from build123d import *

# Parameters (mm, degrees)
SKETCH1_W           = 50
SKETCH1_H           = 57
BOSS_EXTRUDE1_DEPTH = 52
SKETCH2_W           = 18
SKETCH2_H           = 50
CUT_EXTRUDE1_DEPTH  = 52
SKETCH3_W           = 8
SKETCH3_H           = 50
CUT_EXTRUDE2_DEPTH  = 52
SKETCH4_R           = 15
SKETCH4_R_2         = 7
BOSS_EXTRUDE2_DEPTH = 30


with BuildPart() as part:
    # Sketch1 → Boss-Extrude1 (new body)
    with BuildSketch(Plane.XY):
        with Locations((25, 28.5)):
            Rectangle(SKETCH1_W, SKETCH1_H)
    extrude(amount=-BOSS_EXTRUDE1_DEPTH)

    # Sketch2 → Cut-Extrude1 (cut)
    with BuildSketch(Plane.XY):
        with Locations((25, 25)):
            Rectangle(SKETCH2_W, SKETCH2_H)
    extrude(amount=-CUT_EXTRUDE1_DEPTH, mode=Mode.SUBTRACT)

    # Sketch3 → Cut-Extrude2 (cut)
    with BuildSketch(Plane.XY):
        with Locations((46, 32)):
            Rectangle(SKETCH3_W, SKETCH3_H)
        with Locations((4, 32)):
            Rectangle(SKETCH3_W, SKETCH3_H)
    extrude(amount=-CUT_EXTRUDE2_DEPTH, mode=Mode.SUBTRACT)

    # Sketch4 → Boss-Extrude2 (add)
    with BuildSketch(Plane(origin=(42, 0, 0), x_dir=(0, 0, -1), z_dir=(1, 0, 0))):
        with Locations(Location((26, 33, 0), (0, 0, 180))):
            Circle(SKETCH4_R)
        with Locations((26, 33)):
            Circle(SKETCH4_R_2, mode=Mode.SUBTRACT)
    extrude(amount=BOSS_EXTRUDE2_DEPTH)


solid = part.part
Part model, mm, in its own coordinate system. A direction names the side the tool comes from. Round coordinates to 2 decimals unless told otherwise and drop trailing zeros. Loops run counter-clockwise (first coordinate to the right, second up) from the corner with the lowest first, then second, coordinate; pieces in that order, holes last. Notation, with made-up numbers: (46.25, 55.25) - (83.25, 55.25) arc R23 ccw to (83.25, 89.25) - close; hole circle Ø9 at (79.25, 74.5). An arc over 180 degrees is marked (long way). Answer as a JSON object with one key per item and string values.
Item 1: Wall check: L1, parallel to X at y = 47, z = -7; L2, parallel to X at y = 6.5, z = -47.5; L3, parallel to Y at x = 64, z = -26. Give the ranges that are in metal, low to high.
Output:
{"L1": "8 to 16, 34 to 42", "L2": "0 to 16, 34 to 50", "L3": "18 to 26, 40 to 48"}
Item 2: Band-saw the part on A-A on y = 33. List the corners of the cut face in (x, z).
Output:
{"outline": "(8, -52) - (16, -52) - (16, 0) - (8, 0) - close; (34, -52) - (42, -52) - (42, -41) - (72, -41) - (72, -33) - (42, -33) - (42, -19) - (72, -19) - (72, -11) - (42, -11) - (42, 0) - (34, 0) - close"}
Item 3: Tool access for faces 1 (the face through (50, 3, -26)), 2 (the face through (46, 7, -26)), 3 (the face through (34, 25, -26)): list every direction of +Z, -Z, +X, -X, +Y, -Y with a clear straight run to the whole face (end or side of a thin tool).
Output:
{"face 1": "+Z, -Z, +X, -Y", "face 2": "+Z, -Z, +X", "face 3": "+Z, -Z, -Y"}
Item 4: Band-saw the part on D-D on x = 24. List the corners of the cut face in (y, z), plus the area to 3 significant figures.
Output:
{"outline": "(50, -52) - (57, -52) - (57, 0) - (50, 0) - close", "area": "364 mm2"}
Item 5: Band-saw the part on B-B on z = -26. List the corners of the cut face in (x, y).
Output:
{"outline": "(0, 0) - (16, 0) - (16, 50) - (34, 50) - (34, 0) - (50, 0) - (50, 7) - (42, 7) - (42, 18) - (72, 18) - (72, 26) - (42, 26) - (42, 40) - (72, 40) - (72, 48) - (42, 48) - (42, 57) - (8, 57) - (8, 7) - (0, 7) - close"}
Item 6: Pin check, flat tips, straight feed: pin 1 (5 mm diameter, centred on y = 37, z = -42.5, fed in from -X); pin 2 (2 mm diameter, centred on x = 43.5, z = -26.5, fed in from -Y); pin 3 (5 mm diameter, centred on y = 31, z = -46.5, fed in from +X); pin 4 (1 mm diameter, centred on x = 62.5, z = -30, fed in from -Y). Stop position of each tip, or through.
Output:
{"pin 1": "x = 8", "pin 2": "y = 0", "pin 3": "x = 42", "pin 4": "y = 18.41"}
Item 7: Band-saw the part on C-C on y = 17. List the corners of the cut face in (x, z), plus the area to 3 significant figures.
Output:
{"outline": "(8, -52) - (16, -52) - (16, 0) - (8, 0) - close; (34, -52) - (42, -52) - (42, 0) - (34, 0) - close", "area": "832 mm2"}
Item 8: Pull direction Y, two halves, no side cores. Call faces 4 (the face through (42, 0, -26)), 5 (the face through (42, 33, -26)), 6 (the face through (56.79, 39.94, -25.09)), 7 (the face through (25, 57, -26)): pulls with the +Y half, pulls with the -Y half, needs draft (parallel to the pull), parting line crosses it, or undercut.
Output:
{"face 4": "pulls with the -Y half", "face 5": "undercut", "face 6": "undercut", "face 7": "pulls with the +Y half"}
